Input: dimensioned drawing with shaded views. Units: mm. Origin: part minimum x, y, z. Coordinates: 2 decimals unless noted, no trailing zeros. Loops run counter-clockwise (first coordinate to the right, second up) from the corner with the lowest first, then second, coordinate; pieces in that order, holes last.
Item 1: Section query A-A, the plane x = 49.5. Return the cut outline in (y, z), then the cut area to 3 significant figures.
Item 2: Section query B-B, the plane z = 4.5. Return the cut outline in (x, y).
Item 3: Line query: probe 1 along X at (y, z) = (0.2, 5); probe 2 along Z at (x, y) = (102, 0.2); probe 3 along Z at (x, y) = (71, 1.1). Output: solid intervals per line, ascending.
Item 4: Pin query (flat end, axial travel): pin 1 Ø1.5 at (x, y) = (114, 2) entering from -Z; pin 2 Ø1.5 at (y, z) = (1.5, 60.5) entering from -X; pin 3 Ø1.5 at (y, z) = (2, 5) entering from +X. Return the tip coordinate at first contact, or that it passes through.
Item 5: Section query C-C, the plane y = 1.5. State how many separate pieces and enclosed holes the cut face has, then the cut area to 3 significant figures.
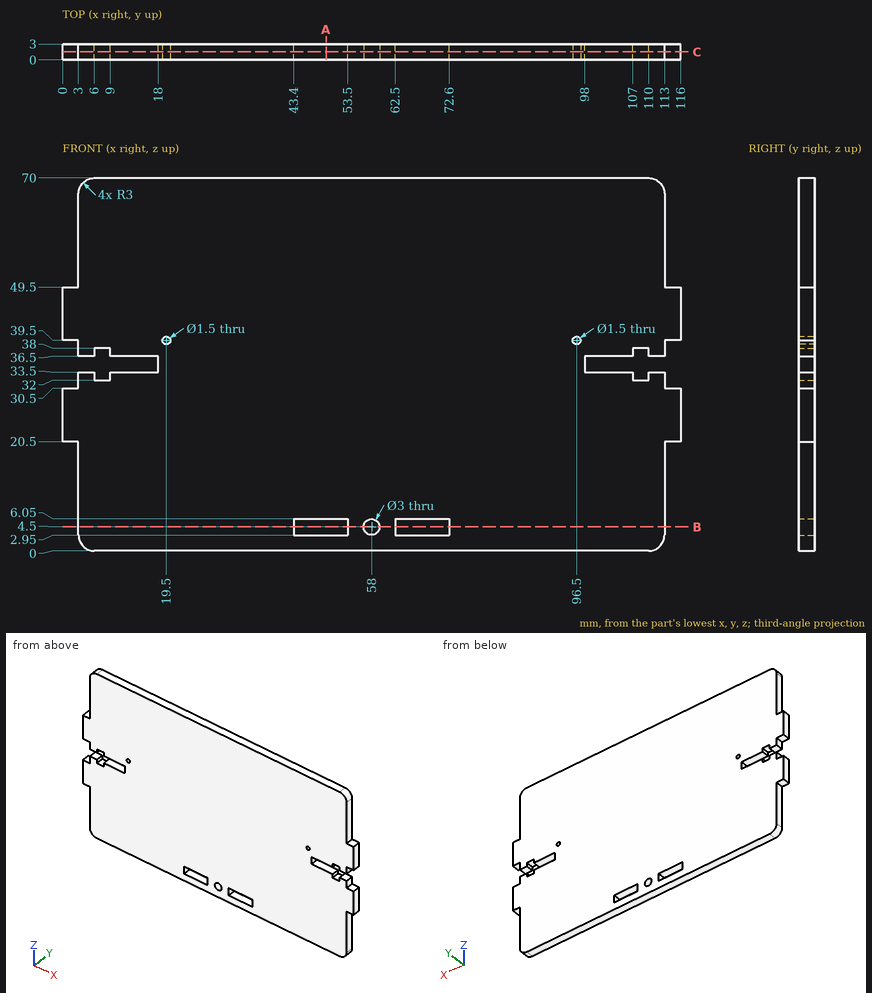
Verdict:
1. outline: (0, 0) - (3, 0) - (3, 2.95) - (0, 2.95) - close; (0, 6.05) - (3, 6.05) - (3, 70) - (0, 70) - close
1. area: 201 mm2
2. outline: (3, 0) - (43.4, 0) - (43.4, 3) - (3, 3) - close; (53.5, 0) - (56.5, 0) - (56.5, 3) - (53.5, 3) - close; (59.5, 0) - (62.5, 0) - (62.5, 3) - (59.5, 3) - close; (72.6, 0) - (113, 0) - (113, 3) - (72.6, 3) - close
3. probe 1: x = 3 to 43.4, 53.5 to 56.59, 59.41 to 62.5, 72.6 to 113
3. probe 2: z = 0 to 33.5, 36.5 to 70
3. probe 3: z = 0 to 2.95, 6.05 to 70
4. pin 1: stops at z = 20.5
4. pin 2: stops at x = 3
4. pin 3: stops at x = 113
5. separate pieces: 1
5. enclosed holes: 5
5. area: 7,630 mm2
